Answer from the drawing. Dimensions are ordinates in mm from the lowest x, y and z of the part. A direction names the side the tool comes from. Coordinates: 2 decimals unless noted, no trailing zeros. Loops run counter-clockwise (first coordinate to the right, second up) from the corner with the lowest first, then second, coordinate; pieces in that order, holes last.
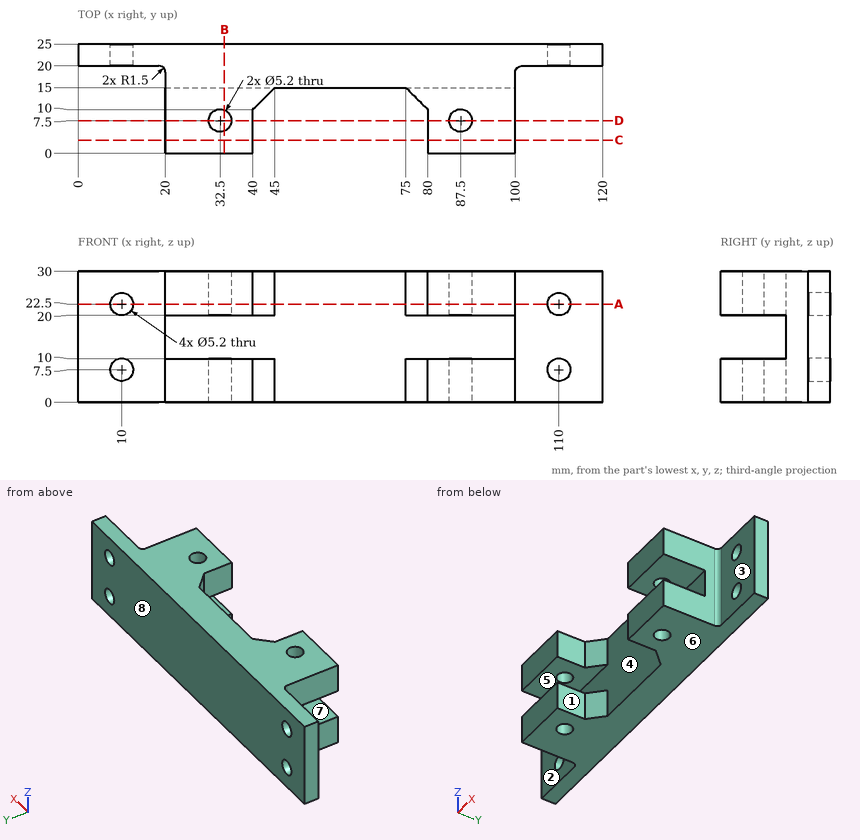
Item 1: A cutting plane is placed at C-C on y = 3. Determine the outline of the cut face in (x, z).
Numbers:
outline: (20, 0) - (40, 0) - (40, 10) - (20, 10) - close; (20, 20) - (40, 20) - (40, 30) - (20, 30) - close; (80, 0) - (100, 0) - (100, 10) - (80, 10) - close; (80, 20) - (100, 20) - (100, 30) - (80, 30) - close
Item 2: Which of the six approach directions +Z, -Z, +X, -X, +Y, -Y give full straight-line access (tool end or side, diameter ignored) to the marked faces 1, 2, 3, 4 and 5?
Numbers:
face 1: +Z, -Z, -Y
face 2: +Z, -Z, -X, -Y
face 3: +Z, -Z, +X, -Y
face 4: -Y
face 5: +X, -X, -Y
Item 3: Given pin 1 (8 mm diameter, centred on y = 5.5, z = 7.5, fed in from -X); pin 2 (3 mm diameter, centred on x = 15.5, z = 5.5, fed in from -Y); pin 3 (9 mm diameter, centred on x = 70, z = 16, fed in from -Y); pin 4 (4.5 mm diameter, centred on x = 87.5, y = 7.5, fed in from -Z), each flat-ended and moving along its own axis, determine where each tip first touches the part or whether it passes through.
Numbers:
pin 1: stops at x = 20
pin 2: stops at y = 20
pin 3: stops at y = 15
pin 4: passes through
Item 4: A cutting plane is placed at D-D on y = 7.5. Give the number of separate pieces and of enclosed holes in the cut face, then the cut area to 3 significant figures.
Numbers:
separate pieces: 8
enclosed holes: 0
area: 592 mm2
Item 5: A cutting plane is placed at A-A on z = 22.5. Determine the outline of the cut face in (x, y).
Numbers:
outline: (0, 20) - (7.4, 20) - (7.4, 25) - (0, 25) - close; (12.6, 20) - (18.5, 20) arc R1.5 cw to (20, 18.5) - (20, 0) - (40, 0) - (40, 10) - (45, 15) - (75, 15) - (80, 10) - (80, 0) - (100, 0) - (100, 18.5) arc R1.5 cw to (101.5, 20) - (107.4, 20) - (107.4, 25) - (12.6, 25) - close; (112.6, 20) - (120, 20) - (120, 25) - (112.6, 25) - close; hole circle Ø5.2 at (32.5, 7.5); hole circle Ø5.2 at (87.5, 7.5)
Item 6: A cutting plane is placed at B-B on x = 33.5. Determine the outline of the cut face in (y, z).
Numbers:
outline: (0, 0) - (5.1, 0) - (5.1, 10) - (0, 10) - close; (0, 20) - (5.1, 20) - (5.1, 30) - (0, 30) - close; (9.9, 0) - (25, 0) - (25, 30) - (9.9, 30) - (9.9, 20) - (15, 20) - (15, 10) - (9.9, 10) - close
Item 7: Determine the mould class of the marked faces 6, 7 and 8 for opening direction Z: released by +Z, released by -Z, zero draft, split by the parting line, or undercut.
Numbers:
face 6: released by -Z
face 7: undercut
face 8: zero draft
Item 8: Find the intervals of material crossed by line 1 along Y through (x, z) = (32.5, 6); line 2 along X through (y, z) = (23.3, 7.5); line 3 along Z through (x, y) = (34, 2.5), in increasing order.
Numbers:
line 1: y = 0 to 4.9, 10.1 to 25
line 2: x = 0 to 7.4, 12.6 to 107.4, 112.6 to 120
line 3: z = 0 to 10, 20 to 30
